from build123d import *
from build123d.topology import SkipClean

# Parameters (mm, degrees)
SKETCH1_R           = 5
SKETCH1_R_2         = 2.6
BOSS_EXTRUDE1_DEPTH = 1.5


with BuildPart() as part:
    # Sketch1 → Boss-Extrude1 (new body)
    # profile 1 of 6: a face of its own
    with SkipClean():  # the faces are left unmerged after this step: merging them gives an invalid solid
        with BuildSketch(Plane.XY):
            Circle(SKETCH1_R)
            Circle(SKETCH1_R_2, mode=Mode.SUBTRACT)
        # profile 2 of 6: a face of its own
        with BuildSketch(Plane.XY):
            with BuildLine():
                Line((-1.967231557, 1.7), (-3.027185929, 1.7))
                Line((-3.027185929, 1.7), (-3.027185929, -1.7))
                Line((-3.027185929, -1.7), (-1.967231557, -1.7))
                ThreePointArc((-1.967231557, -1.7), (-2.6, 0), (-1.967231557, 1.7))
            make_face()
        # profile 3 of 6: a face of its own
        with BuildSketch(Plane.XY):
            with BuildLine():
                ThreePointArc((1.967231557, 1.7), (0, 2.6), (-1.967231557, 1.7))
                Line((-1.967231557, 1.7), (1.967231557, 1.7))
            make_face()
        # profile 4 of 6: a face of its own
        with BuildSketch(Plane.XY):
            with BuildLine():
                Line((3.027185929, 1.7), (1.967231557, 1.7))
                ThreePointArc((1.967231557, 1.7), (2.436678277, 0.906972423), (2.6, 0))
                ThreePointArc((2.6, 0), (2.436678277, -0.906972423), (1.967231557, -1.7))
                Line((1.967231557, -1.7), (3.027185929, -1.7))
                Line((3.027185929, -1.7), (3.027185929, 1.7))
            make_face()
        # profile 5 of 6: a face of its own
        with BuildSketch(Plane.XY):
            with BuildLine():
                Line((1.967231557, -1.7), (-1.967231557, -1.7))
                ThreePointArc((-1.967231557, -1.7), (0, -2.6), (1.967231557, -1.7))
            make_face()
        # profile 6 of 6: a face of its own
        with BuildSketch(Plane.XY):
            with BuildLine():
                Line((0, 6.272587449), (-1.733646509, 4.6898262))
                ThreePointArc((-1.733646509, 4.6898262), (-0.067970608, 4.999537978), (1.6055094, 4.735223286))
                Line((1.6055094, 4.735223286), (0, 6.272587449))
            make_face()
        extrude(amount=BOSS_EXTRUDE1_DEPTH)


solid = part.part
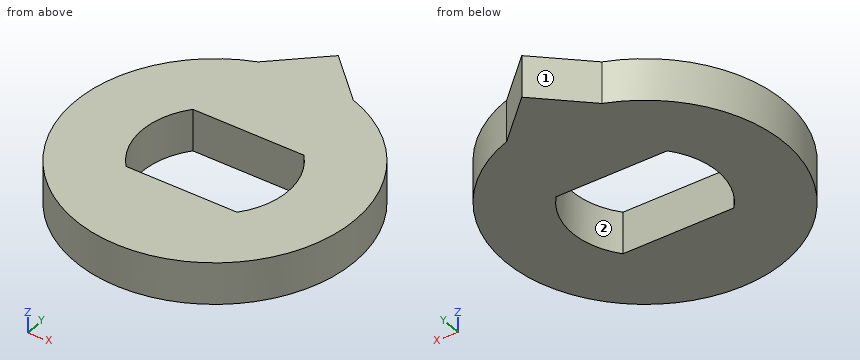
For this review, take the finished solid that the model builds, in its own axes (mm). Face numbers are marked on the shaded views. A direction names the side the tool comes from. Give positions to 0.01 mm unless a question says otherwise; leave off trailing zeros. Loops run counter-clockwise (first coordinate to the right, second up) from the corner with the lowest first, then second, coordinate; pieces in that order, holes last.
Item 1: Take a section at C-C, the plane x = -2.25. State the section outline as (y, z) points.
Item 2: Tool access review of the marked faces 1 and 2: name each direction out of +Z, -Z, +X, -X, +Y, -Y from which nothing blocks a thin tool from reaching the whole face with its end or side.
Item 3: Take a section at A-A, the plane z = 1.3. State the section outline as (x, y) points.
Item 4: For line 1 along Y through (x, z) = (-0.75, 0.45); line 2 along Y through (x, z) = (-1, 0.55); line 3 along X through (y, z) = (0.75, 0.35), list the stretches that pass through material, from the lowest coordinate up.
Item 5: Take a section at B-B, the plane y = 0. State the section outline as (x, z) points, and give its area (3 significant figures).
Item 6: Take a section at D-D, the plane y = 4. State the section outline as (x, z) points, and give its area (3 significant figures).
Calculated:
1. outline: (-4.47, 0) - (-1.3, 0) - (-1.3, 1.5) - (-4.47, 1.5) - close; (1.3, 0) - (4.47, 0) - (4.47, 1.5) - (1.3, 1.5) - close
2. face 1: +Z, -Z, -X, +Y
2. face 2: +Z, -Z
3. outline: (-1.73, 4.69) arc R5 ccw (long way) to (1.61, 4.74) - (0, 6.27) - close; hole (-1.97, -1.7) - (1.97, -1.7) arc R2.6 ccw to (1.97, 1.7) - (-1.97, 1.7) arc R2.6 ccw to start
4. line 1: y = -4.94 to -1.7, 1.7 to 5.59
4. line 2: y = -4.9 to -1.7, 1.7 to 5.36
4. line 3: x = -4.94 to -2.49, 2.49 to 4.94
5. outline: (-5, 0) - (-2.6, 0) - (-2.6, 1.5) - (-5, 1.5) - close; (2.6, 0) - (5, 0) - (5, 1.5) - (2.6, 1.5) - close
5. area: 7.20 mm2
6. outline: (-3, 0) - (3, 0) - (3, 1.5) - (-3, 1.5) - close
6. area: 9.00 mm2
